Autodesk Inventor part; units mm, degrees
ref_plane "YZ Plane" through (0, 0, 0) normal (1, 0, 0) x (0, 1, 0)
ref_plane "XZ Plane" through (0, 0, 0) normal (0, 1, 0) x (-1, 0, 0)
ref_plane "XY Plane" through (0, 0, 0) normal (0, 0, 1) x (1, 0, 0)
sketch "Sketch1" plane through (0, 0, 0) normal (0, 1, 0) x (-1, 0, 0)
  line L0 (12.35, 8.5) -> (-12.35, 8.5)
  line L1 (-12.35, 8.5) -> (-12.35, -8.5)
  line L2 (-12.35, -8.5) -> (12.35, -8.5)
  line L3 (12.35, -8.5) -> (12.35, 8.5)
  line L4 (12.35, 8.5) -> (-12.35, -8.5) construction
  line L5 (-12.35, 8.5) -> (12.35, -8.5) construction
  point P0 (0, 0)
  dimension "d0" = 24.7
  dimension "d1" = 17
extrude "Extrusion1" add sketch "Sketch1" along normal blind 10
sketch "Sketch2" plane through (0, 10, 0) normal (0, 1, 0) x (1, 0, 0)
  line L0 (-12.35, 8.1) -> (12.35, 8.1)
  line L1 (12.35, 8.1) -> (12.35, -8.1)
  line L2 (12.35, -8.1) -> (-12.35, -8.1)
  line L3 (-12.35, -8.1) -> (-12.35, 8.1)
  line L4 (-12.35, 8.1) -> (12.35, -8.1) construction
  line L5 (12.35, 8.1) -> (-12.35, -8.1) construction
  point P0 (0, 0)
  dimension "d4" = 24.7
  dimension "d5" = 16.2
extrude "Extrusion2" cut sketch "Sketch2" against normal blind 9
sketch "Sketch3" plane through (0, 0, 0) normal (0, -1, 0) x (1, 0, 0)
  line L0 (-12.35, -8.5) -> (-12.35, 8.5)
  line L1 (12.35, 8.5) -> (12.35, -8.5)
  line L2 (-12.35, 0) -> (-9.35, 0)
  circle A0 centre (-9.35, 0) radius 1.5
  line L3 (12.35, 0) -> (9.35, 0)
  circle A1 centre (9.35, 0) radius 1.5
  point P0 (0, 0)
  dimension "d8" = 3
  dimension "d9" = 3
  dimension "d10" = 3
  dimension "d11" = 3
extrude "Extrusion3" cut sketch "Sketch3" against normal blind 1
sketch "Sketch4" plane through (-12.35, 0, -8.5) normal (-1, 0, 0) x (0, 0, 1)
  line L0 (0.4, 1) -> (0.4, 10)
  line L1 (0, 10) -> (0.4, 10)
  line L2 (0, 0) -> (0, 10)
  line L3 (0, 0) -> (17, 0)
  line L4 (17, 0) -> (17, 10)
  line L5 (16.6, 10) -> (17, 10)
  line L6 (16.6, 10) -> (16.6, 1)
  line L7 (16.6, 1) -> (0.4, 1)
  point P0 (8.5, 0)
extrude "Extrusion4" add sketch "Sketch4" along normal blind 2
sketch "Sketch5" plane through (-14.35, 0, -8.5) normal (-1, 0, 0) x (0, 0, 1)
  line L0 (0.4, 1) -> (0.4, 10)
  line L1 (0.4, 10) -> (0, 10)
  line L2 (0, 10) -> (0, 0)
  line L3 (0, 0) -> (17, 0)
  line L4 (17, 0) -> (17, 10)
  line L5 (17, 10) -> (16.6, 10)
  line L6 (16.6, 10) -> (16.6, 1)
  line L7 (16.6, 1) -> (0.4, 1)
  point P0 (8.5, 0)
extrude "Extrusion5" cut sketch "Sketch5" against normal blind 0.2
sketch "Sketch6" plane through (0, 0, 0) normal (0, -1, 0) x (1, 0, 0)
  line L0 (-14.15, 8.5) -> (-14.15, -8.5)
  line L1 (-14.15, 8.5) -> (12.35, 8.5)
  circle A0 centre (-9.35, 0) radius 1.5
  line L2 (-14.15, 0) -> (-12.15, 0)
  line L3 (-12.15, 0) -> (-10.15, 0)
  line L4 (-10.15, 0) -> (-7.15, 0)
  point P0 (0, 0)
  dimension "d18" = 2
  dimension "d19" = 2
  dimension "d20" = 3
extrude "Extrusion6" add sketch "Sketch6" against normal blind 1
sketch "Sketch7" plane through (0, 0, 0) normal (0, -1, 0) x (1, 0, 0)
  line L0 (-14.15, 8.5) -> (-14.15, -8.5)
  line L1 (-14.15, 8.5) -> (12.35, 8.5)
  line L2 (-14.15, 0) -> (-10.85, 0)
  line L3 (-10.85, 0) -> (-7.85, 0)
  circle A0 centre (-7.85, 0) radius 1.5
  point P0 (0, 0)
  dimension "d29" = 3.3
  dimension "d30" = 3
  dimension "d31" = 3
extrude "Extrusion7" cut sketch "Sketch7" against normal blind 1
sketch "Sketch8" plane through (0, 1, 0) normal (0, 1, 0) x (1, 0, 0)
  circle A0 centre (-7.85, 0) radius 1.5
  circle A1 centre (9.35, 0) radius 1.5
  circle A2 centre (9.35, 0) radius 0.05
  circle A3 centre (-7.85, 0) radius 0.05
  point P0 (0, 0)
  dimension "d34" = 0.1
  dimension "d35" = 0.1
extrude "Extrusion8" add sketch "Sketch8" against normal blind 1
properties part number "kolejnicka_ruka_sablona"
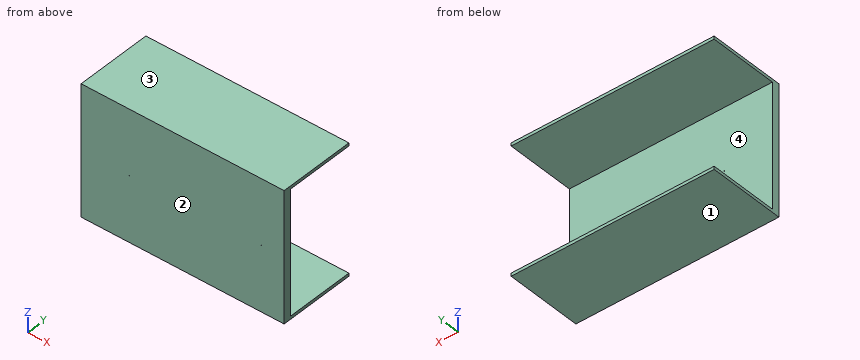
CAD build for the part. Positions are in the model's coordinates, mm. Face numbers are marked on the shaded views. Give positions to 0.01 mm unless a question says otherwise; leave off trailing zeros. Write each loop counter-clockwise with the first axis right and the second up, starting at its lowest first coordinate (ties: lowest second). Pieces come first, ordered by that corner, then holes. Notation, with made-up numbers: M -6.75,1.5 L -0.75,1.5 A12 ccw -0.75,13.5 Z; hole C -7,-17.5 d4. An arc over 180 degrees is marked long. Put each result on its own line as item: value. Start each with the question number.
(1) Band-saw the part on C-C, the plane z = 0.5. Write the cut outline in (x, y).
(2) Probe L1, parallel to Z at x = 2.25, y = 5.75; L2, parallel to Y at x = -5.25, z = 7.5. List the from-to ranges inside material, lowest first.
(3) Flat gauge pin, fed straight in: pin 1 Ø1.5 at (y, z) = (8, -6) entering from +X. Where does the tip first touch, or does it go through?
(4) Band-saw the part on B-B, the plane x = 0. Write the cut outline in (y, z), and give its area (3 significant figures).
(5) Mould opens along Z. For the marked faces 1, 2, 3 and 4 say: +Z half, -Z half, draft (parallel to the pull), parting line (faces both ways), or undercut.
(6) Band-saw the part on A-A, the plane y = 8.25. Write the cut outline in (x, z), and give its area (3 significant figures).
Response values:
1. outline: M -14.15,0 L 12.35,0 L 12.35,1 L -14.15,1 Z
2. L1: z = -8.5 to -8.1, 8.1 to 8.5
2. L2: y = 0 to 1
3. pin 1: passes through
4. outline: M 0,-8.5 L 10,-8.5 L 10,-8.1 L 1,-8.1 L 1,8.1 L 10,8.1 L 10,8.5 L 0,8.5 Z
4. area: 24.2 mm2
5. face 1: -Z half
5. face 2: draft
5. face 3: +Z half
5. face 4: undercut
6. outline: M -14.15,-8.5 L 12.35,-8.5 L 12.35,-8.1 L -14.15,-8.1 Z; M -14.15,8.1 L 12.35,8.1 L 12.35,8.5 L -14.15,8.5 Z
6. area: 21.2 mm2
